For this review, take the finished solid that the model builds, in its own axes (mm). Face numbers are marked on the shaded views. A direction names the side the tool comes from. Give positions to 0.01 mm unless a question says otherwise; leave off trailing zeros. Write each loop counter-clockwise with the first axis right and the second up, starting at its lowest first coordinate (ties: lowest second). Pieces come first, ordered by that corner, then holes.
Q1. We need section B-B (z = 17.5). Write out the cut boundary in (x, y) (3 decimals), then the cut area to 3 significant figures.
Q2. Insertion check: P1, Ø10, axis at x = 12.5, z = -43.5, coming from the -Y side; P2, Ø2, axis at x = 0.5, y = 24.5, coming from the +Z side; P3, Ø18, axis at x = -1, y = 1.5, coming from the +Z side. Each pin has a flat end and moves straight along its axis. Give the tip position at first contact, or say it passes through.
Q3. We need section C-C (y = 61). Write out the cut boundary in (x, z).
Q4. We need section A-A (x = -18). Write out the cut boundary in (y, z), then the cut area to 3 significant figures.
Q5. Machinability: for the marked faces 1, 2 and 3, which of the approach directions +Z, -Z, +X, -X, +Y, -Y give a long, thin tool a straight path to every point of the face, cutting with its end or side? Answer none if there is none.
Q6. For line 1 (Y direction, x = -12, z = 50.5); line 2 (Y direction, x = -16, z = 45); line 3 (Y direction, x = -5, z = -37), list the stretches that pass through material, from the lowest coordinate up.
Q7. Mouldability with a two-part tool opening along Y and no side actions: class the marked faces 4, 5 and 6 as released by +Y, released by -Y, zero draft, split by the parting line, or undercut.
```python
from build123d import *

# Parameters (mm, degrees)
F1_DEPTH = 30


with BuildPart() as f1:
    # F0 (on Right) → F1 (new body, symmetric)
    with BuildSketch(Plane.YZ):
        with BuildLine():
            ThreePointArc((-76.238519, -57.397258), (-78.618579, -56.223542), (-79.136297, -53.620801))
            Line((-79.136297, -53.620801), (-74.124065, -34.914896))
            Line((-74.124065, -34.914896), (-77.987768, -33.87962))
            Line((-77.987768, -33.87962), (-83, -52.585524))
            ThreePointArc((-83, -52.585524), (-81.791993, -58.658588), (-76.238519, -61.397258))
            Line((-76.238519, -61.397258), (23.690404, -61.397258))
            ThreePointArc((23.690404, -61.397258), (51.859532, -52.954337), (70.740883, -30.409332))
            ThreePointArc((70.740883, -30.409332), (73.50453, 22.936522), (40.893049, 65.243839))
            ThreePointArc((40.893049, 65.243839), (23.901637, 67.952883), (10.156762, 57.602742))
            Line((10.156762, 57.602742), (-56.238519, -57.397258))
            Line((-56.238519, -57.397258), (-76.238519, -57.397258))
        make_face()
        with BuildLine():
            ThreePointArc((13.620863, 55.602742), (24.86667, 64.071039), (38.768735, 61.854549))
            ThreePointArc((38.768735, 61.854549), (69.686113, 21.745014), (67.066032, -28.829626))
            ThreePointArc((67.066032, -28.829626), (49.659399, -49.613767), (23.690404, -57.397258))
            Line((23.690404, -57.397258), (-51.619717, -57.397258))
            Line((-51.619717, -57.397258), (13.620863, 55.602742))
        make_face(mode=Mode.SUBTRACT)
    extrude(amount=F1_DEPTH, both=True)


solid = f1.part
```
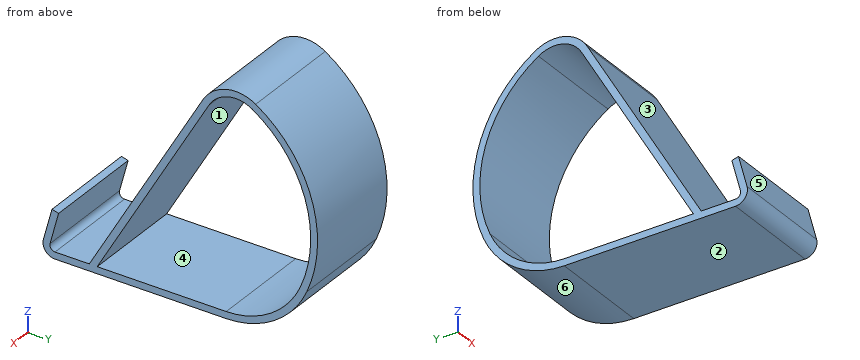
Computed:
1. outline: (-30, -12.997) - (30, -12.997) - (30, -8.378) - (-30, -8.378) - close; (-30, 70.871) - (30, 70.871) - (30, 74.985) - (-30, 74.985) - close
1. area: 524 mm2
2. P1: stops at y = -81.91
2. P2: stops at z = 68.29
2. P3: stops at z = 58.18
3. outline: (-30, -45.27) - (30, -45.27) - (30, -39.12) - (-30, -39.12) - close; (-30, 40.1) - (30, 40.1) - (30, 46.99) - (-30, 46.99) - close
4. outline: (-83, -52.59) arc R7 ccw to (-76.24, -61.4) - (23.69, -61.4) arc R51.21 ccw to (70.74, -30.41) arc R77 ccw to (40.89, 65.24) arc R22 ccw to (10.16, 57.6) - (-56.24, -57.4) - (-76.24, -57.4) arc R3 cw to (-79.14, -53.62) - (-74.12, -34.91) - (-77.99, -33.88) - close; hole (-51.62, -57.4) - (23.69, -57.4) arc R47.21 ccw to (67.07, -28.83) arc R73 ccw to (38.77, 61.85) arc R18 ccw to (13.62, 55.6) - close
4. area: 1,820 mm2
5. face 1: +X, -X
5. face 2: -Z, +X, -X, +Y, -Y
5. face 3: +Z, +X, -X
6. line 1: y = 6.06 to 10.67, 52.71 to 58.13
6. line 2: y = 2.88 to 7.5, 57.48 to 62.48
6. line 3: y = -78.82 to -74.68, -44.46 to -39.84, 62.55 to 67.32
7. face 4: undercut
7. face 5: released by -Y
7. face 6: released by +Y
